```python
from build123d import *

# Parameters (mm, degrees)
EXTRUSION1_DEPTH = 80
ESQUISSE2_R      = 1.5
ESQUISSE2_W      = 2.5
ESQUISSE2_H      = 20
EXTRUSION2_DEPTH = 10
ESQUISSE3_R      = 2
EXTRUSION3_DEPTH = 88.508383337


with BuildPart() as part:
    # Esquisse1 → Extrusion1 (new body)
    with BuildSketch(Plane.XY):
        Polygon((-29.286808535, 30.629808714), (-29.286808535, 10.629808714), (-9.286808535, 10.629808714), (-9.286808535, 12.129808714), (-27.786808535, 12.129808714), (-27.786808535, 29.129808714), (-9.286808535, 29.129808714), (-9.286808535, 30.629808714), align=None)
    extrude(amount=EXTRUSION1_DEPTH)

    # Esquisse2 → Extrusion2 (cut)
    with BuildSketch(Plane.XZ.offset(-10.629808714)):
        with Locations(Location((-14.286808535, 74, 0), (0, 0, 270))):
            Circle(ESQUISSE2_R)
        with Locations(Location((-24.286808535, 74, 0), (0, 0, 270))):
            Circle(ESQUISSE2_R)
        with Locations(Location((-14.286808535, 16, 0), (0, 0, 270))):
            Circle(ESQUISSE2_R)
        with Locations(Location((-24.286808535, 10, 0), (0, 0, 270))):
            Circle(ESQUISSE2_R)
        with Locations((-10.536808535, 40)):
            Rectangle(ESQUISSE2_W, ESQUISSE2_H)
    extrude(amount=-EXTRUSION2_DEPTH, mode=Mode.SUBTRACT)

    # Esquisse3 → Extrusion3 (cut, through all)
    with BuildSketch(Plane.XZ.offset(-10.629808714)):
        with Locations(Location((-19.286808535, 40, 0), (0, 0, 270))):
            Circle(ESQUISSE3_R)
    extrude(amount=-EXTRUSION3_DEPTH, mode=Mode.SUBTRACT)


solid = part.part
```
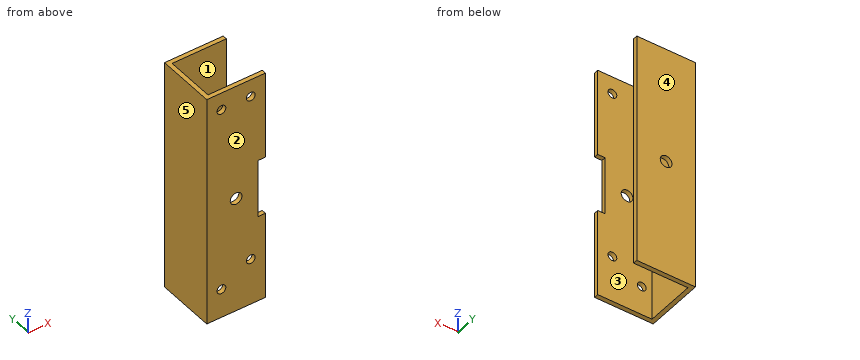
Geometry check sheet. Reference: the model listing, model coordinates, mm. Face numbers are marked on the shaded views. A direction names the side the tool comes from. Coordinates: 2 decimals unless noted, no trailing zeros. Write each loop counter-clockwise with the first axis right and the second up, starting at its lowest first coordinate (ties: lowest second). Pieces come first, ordered by that corner, then holes. Notation, with made-up numbers: M 41.5,-31.75 L 63.5,-31.75 A12 ccw 63.5,-22.75 Z; hole C -18.75,-39 d4. An arc over 180 degrees is marked long. Use one line per item in the form item = value. Start each with the question number.
1) Go/stop test with flat-tipped pins: pin 1 Ø1.6 at (y, z) = (11, 37) entering from +X; pin 2 Ø2.5 at (x, z) = (-14.29, 74) entering from -Y; pin 3 Ø8.5 at (y, z) = (21.5, 52) entering from +X. Record where each tip stops, or that it passes through.
2) Release check for a two-part mould opening along Y. For the marked faces 3, 4 and 5 record: pulls with the +Y half, pulls with the -Y half, needs draft (parallel to the pull), parting line crosses it, or undercut.
3) Section check B-B on z = 10. Enter the section's corners in (x, y).
4) Section check C-C on x = -18.5. Enter the section's corners in (y, z), and give its area (3 significant figures).
5) Section check A-A on z = 40. Enter the section's corners in (x, y).
6) Thickness scan on probe 1 along Y at (x, z) = (-13.25, 70); probe 2 along X at (y, z) = (30.3, 40); probe 3 along X at (y, z) = (11.65, 10). Record the ranges inside material, lowest first. Write a range as from..to.
7) Section check D-D on z = 64. Enter the section's corners in (x, y).
8) Set-up check for the marked faces 1 and 2: record each of +Z, -Z, +X, -X, +Y, -Y from which the full face is reachable in a straight line by a thin tool's end or side.
Responses:
q1.pin_1 = -11.79
q1.pin_2 = 29.13
q1.pin_3 = -27.79
q2.face_3 = undercut
q2.face_4 = pulls with the +Y half
q2.face_5 = needs draft
q3.outline = M -29.29,10.63 L -25.79,10.63 L -25.79,12.13 L -27.79,12.13 L -27.79,29.13 L -9.29,29.13 L -9.29,30.63 L -29.29,30.63 Z; M -22.79,10.63 L -9.29,10.63 L -9.29,12.13 L -22.79,12.13 Z
q4.outline = M 10.63,0 L 12.13,0 L 12.13,38.16 L 10.63,38.16 Z; M 10.63,41.84 L 12.13,41.84 L 12.13,80 L 10.63,80 Z; M 29.13,0 L 30.63,0 L 30.63,38.16 L 29.13,38.16 Z; M 29.13,41.84 L 30.63,41.84 L 30.63,80 L 29.13,80 Z
q4.area = 229 mm2
q5.outline = M -29.29,10.63 L -21.29,10.63 L -21.29,12.13 L -27.79,12.13 L -27.79,29.13 L -21.29,29.13 L -21.29,30.63 L -29.29,30.63 Z; M -17.29,10.63 L -11.79,10.63 L -11.79,12.13 L -17.29,12.13 Z; M -17.29,29.13 L -9.29,29.13 L -9.29,30.63 L -17.29,30.63 Z
q6.probe_1 = 10.63..12.13, 29.13..30.63
q6.probe_2 = -29.29..-21.29, -17.29..-9.29
q6.probe_3 = -29.29..-25.79, -22.79..-9.29
q7.outline = M -29.29,10.63 L -9.29,10.63 L -9.29,12.13 L -27.79,12.13 L -27.79,29.13 L -9.29,29.13 L -9.29,30.63 L -29.29,30.63 Z
q8.face_1 = +Z, -Z, +X
q8.face_2 = +Z, -Z, +X, -X, -Y
